Geometry check sheet. Reference: the model listing, model coordinates, mm. A direction names the side the tool comes from. Coordinates: 2 decimals unless noted, no trailing zeros. Order: outer loops, then holes, each group sorted by start corner. A loop starts at its lowest first (then second) coordinate and runs counter-clockwise, first axis right, second up. Notation, with made-up numbers: (0.25, 80.5) - (43.25, 80.5) arc R27 cw to (43.25, 111.5) - close; hole circle Ø10 at (62.5, 61.5). An arc over 180 degrees is marked (long way). Use CSV: the item, a comma, the result in double quotes. Start each with the question number.
1) Tool access check on faces 1 (the cylindrical face through (18.257, 6.056, -6.604)), 2 (the flat face through (34, 8, 1)), 3 (the flat face through (10, 10, 2)). Record the directions out of +Z, -Z, +X, -X, +Y, -Y that give a thin tool (end or side, any length) a straight path to the whole face; none if there is none.
2) Sectioned sample at A-A, the plane z = -11.55. Record the cut outline in (x, y), and give its area (3 significant figures).
3) Draft check along Z on faces 4 (the cylindrical face through (42.581, 6.056, -13.544)), 5 (the flat face through (34, 8, 22.05)), 6 (the flat face through (33, 10, -2)). Enter one of: released by +Z, released by -Z, zero draft, split by the parting line, or undercut.
4) Sectioned sample at C-C, the plane z = 3.5. Record the cut outline in (x, y), and give its area (3 significant figures).
5) Depth check by flat-ended pin: P1, Ø14.5, axis at x = 11, z = -7.5, coming from the +Y side; P2, Ø5, axis at y = 30, z = -2.5, coming from the -X side; P3, Ø24, axis at x = 33.6, z = -11.55, coming from the +Y side. Enter the tip coordinate at first touch or a pass-through.
6) Sectioned sample at D-D, the plane y = 59.5. Record the cut outline in (x, z), and give its area (4 significant figures).
7) Sectioned sample at B-B, the plane x = 33.6. Record the cut outline in (y, z), and give its area (3 significant figures).
8) Thickness scan on probe 1 along X at (y, z) = (4.5, 11.55); probe 2 along X at (y, z) = (1.05, -11.55); probe 3 along Z at (x, y) = (42, 8). Record the ranges inside material, lowest first. Write a range as [from, to].
from build123d import *

# Parameters (mm, degrees)
SKETCH1_W               = 44.1
SKETCH1_H               = 44.1
BOSS_EXTRUDE1_DEPTH     = 10
SKETCH2_R               = 9.2
CUT_EXTRUDE1_DEPTH      = 8
SKETCH5_R               = 6.65
CUT_EXTRUDE4_DEPTH      = 50.9501001
MIRROR2_COPY_1_SKETCH_R = 9.2
MIRROR2_COPY_1_DEPTH    = 8
MIRROR2_COPY_2_SKETCH_R = 6.65
MIRROR2_COPY_2_DEPTH    = 50.9501001
CUT_EXTRUDE3_DEPTH      = 5
SKETCH6_W               = 44.1
SKETCH6_H               = 10
BOSS_EXTRUDE2_DEPTH     = 5
SKETCH7_W               = 5
SKETCH7_H               = 44.1
BOSS_EXTRUDE3_DEPTH     = 53.9


with BuildPart() as part:
    # Sketch1 → Boss-Extrude1 (new body)
    with BuildSketch(Plane(origin=(0, 0, 0), x_dir=(1, 0, 0), z_dir=(0, 1, 0))):
        with Locations((22.05, 0)):
            Rectangle(SKETCH1_W, SKETCH1_H)
    extrude(amount=BOSS_EXTRUDE1_DEPTH)

    # Sketch2 → Cut-Extrude1 (cut)
    with BuildSketch(Plane(origin=(0, 10, 0), x_dir=(1, 0, 0), z_dir=(0, 1, 0))):
        with Locations(Location((10.5, 11.55, 0), (0, 0, 270))):
            Circle(SKETCH2_R)
    cut_extrude1 = extrude(amount=-CUT_EXTRUDE1_DEPTH, mode=Mode.SUBTRACT)

    # Sketch5 → Cut-Extrude4 (cut, through all)
    with BuildSketch(Plane(origin=(0, 2, 0), x_dir=(1, 0, 0), z_dir=(0, 1, 0))):
        with Locations(Location((10.5, 11.55, 0), (0, 0, 270))):
            Circle(SKETCH5_R)
    cut_extrude4 = extrude(amount=-CUT_EXTRUDE4_DEPTH, mode=Mode.SUBTRACT)

    # Mirror1: Cut-Extrude1, Cut-Extrude4 across plane
    add(cut_extrude1.mirror(Plane.XY), mode=Mode.SUBTRACT)
    add(cut_extrude4.mirror(Plane.XY), mode=Mode.SUBTRACT)

    # Mirror2: Cut-Extrude1, Cut-Extrude4 across plane
    add(cut_extrude1.mirror(Plane(origin=(22.05, 0, 0), x_dir=(0, 0, 1), z_dir=(1, 0, 0))), mode=Mode.SUBTRACT)
    add(cut_extrude4.mirror(Plane(origin=(22.05, 0, 0), x_dir=(0, 0, 1), z_dir=(1, 0, 0))), mode=Mode.SUBTRACT)

    # Mirror2 copy 1 sketch → Mirror2 copy 1 (cut)
    with BuildSketch(Plane(origin=(44.1, 10, 0), x_dir=(-1, 0, 0), z_dir=(0, 1, 0))):
        with Locations(Location((10.5, 11.55, 0), (0, 0, 270))):
            Circle(MIRROR2_COPY_1_SKETCH_R)
    extrude(amount=-MIRROR2_COPY_1_DEPTH, mode=Mode.SUBTRACT)

    # Mirror2 copy 2 sketch → Mirror2 copy 2 (cut, through all)
    with BuildSketch(Plane(origin=(44.1, 2, 0), x_dir=(-1, 0, 0), z_dir=(0, 1, 0))):
        with Locations(Location((10.5, 11.55, 0), (0, 0, 270))):
            Circle(MIRROR2_COPY_2_SKETCH_R)
    extrude(amount=-MIRROR2_COPY_2_DEPTH, mode=Mode.SUBTRACT)

    # Sketch4 → Cut-Extrude3 (cut)
    with BuildSketch(Plane(origin=(0, 10, 0), x_dir=(1, 0, 0), z_dir=(0, 1, 0))):
        Polygon((21.05, 22.05), (23.05, 22.05), (23.05, 1), (46.251393124, 1), (46.251393124, -1), (23.05, -1), (23.05, -23.362709558), (21.05, -23.362709558), (21.05, -1), (0, -1), (0, 1), (21.05, 1), align=None)
    extrude(amount=-CUT_EXTRUDE3_DEPTH, mode=Mode.SUBTRACT)

    # Sketch6 → Boss-Extrude2 (add)
    with BuildSketch(Plane(origin=(44.1, 0, 0), x_dir=(0, 0, -1), z_dir=(1, 0, 0))):
        with Locations((0, 5)):
            Rectangle(SKETCH6_W, SKETCH6_H)
    extrude(amount=BOSS_EXTRUDE2_DEPTH)

    # Sketch7 → Boss-Extrude3 (add)
    with BuildSketch(Plane(origin=(0, 10, 0), x_dir=(1, 0, 0), z_dir=(0, 1, 0))):
        with Locations((46.6, 0)):
            Rectangle(SKETCH7_W, SKETCH7_H)
    extrude(amount=BOSS_EXTRUDE3_DEPTH)


solid = part.part
Evaluation:
1,face 1,"+Y"
1,face 2,"-X, +Y"
1,face 3,"+Z, -Z, -X, +Y"
2,outline,"(0, 0) - (3.85, 0) - (3.85, 2) - (1.3, 2) - (1.3, 10) - (0, 10) - close; (17.15, 0) - (26.95, 0) - (26.95, 2) - (24.4, 2) - (24.4, 10) - (23.05, 10) - (23.05, 5) - (21.05, 5) - (21.05, 10) - (19.7, 10) - (19.7, 2) - (17.15, 2) - close; (40.25, 0) - (49.1, 0) - (49.1, 63.9) - (44.1, 63.9) - (44.1, 10) - (42.8, 10) - (42.8, 2) - (40.25, 2) - close"
2,area,"403 mm²"
3,face 4,"undercut"
3,face 5,"released by +Z"
3,face 6,"zero draft"
4,outline,"(0, 0) - (49.1, 0) - (49.1, 63.9) - (44.1, 63.9) - (44.1, 10) - (38.05, 10) - (38.05, 2) - (29.15, 2) - (29.15, 10) - (23.05, 10) - (23.05, 5) - (21.05, 5) - (21.05, 10) - (14.95, 10) - (14.95, 2) - (6.05, 2) - (6.05, 10) - (0, 10) - close"
4,area,"608 mm²"
5,P1,"y = 10"
5,P2,"x = 44.1"
5,P3,"y = 63.9"
6,outline,"(44.1, -22.05) - (49.1, -22.05) - (49.1, 22.05) - (44.1, 22.05) - close"
6,area,"220.5 mm²"
7,outline,"(0, -22.05) - (10, -22.05) - (10, -20.75) - (2, -20.75) - (2, -18.2) - (0, -18.2) - close; (0, -4.9) - (2, -4.9) - (2, -2.35) - (10, -2.35) - (10, -1) - (5, -1) - (5, 1) - (10, 1) - (10, 2.35) - (2, 2.35) - (2, 4.9) - (0, 4.9) - close; (0, 18.2) - (2, 18.2) - (2, 20.75) - (10, 20.75) - (10, 22.05) - (0, 22.05) - close"
7,area,"83.4 mm²"
8,probe 1,"[0, 1.3], [19.7, 24.4], [42.8, 49.1]"
8,probe 2,"[0, 3.85], [17.15, 26.95], [40.25, 49.1]"
8,probe 3,"[-22.05, -15.3], [-7.8, -1], [1, 7.8], [15.3, 22.05]"
